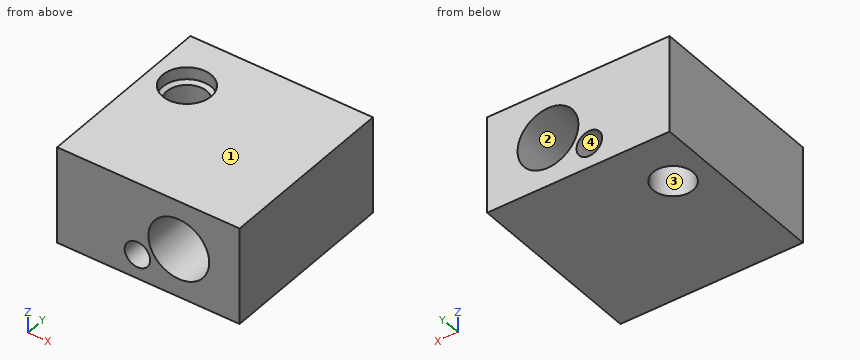
```python
from build123d import *

# Parameters (mm, degrees)
SKETCH1_W                    = 15
SKETCH1_H                    = 15
SKETCH1_R                    = 1.65
BOSS_EXTRUDE1_DEPTH          = 8
SKETCH2_R                    = 2.5
CUT_EXTRUDE1_DEPTH           = 16
SKETCH3_R                    = 1.05
CUT_EXTRUDE2_DEPTH           = 16
F_4_0_4_DIAMETER_HOLE1_D     = 4
F_4_0_4_DIAMETER_HOLE1_DEPTH = 1
F_4_0_4_DIAMETER_HOLE1_TIP   = 1.201721238


with BuildPart() as part:
    # Sketch1 → Boss-Extrude1 (new body)
    with BuildSketch(Plane.XY):
        with Locations((4.5, -3)):
            Rectangle(SKETCH1_W, SKETCH1_H)
        Circle(SKETCH1_R, mode=Mode.SUBTRACT)
    extrude(amount=BOSS_EXTRUDE1_DEPTH)

    # Sketch2 → Cut-Extrude1 (cut, through all)
    with BuildSketch(Plane.XZ.offset(10.5)):
        with Locations((7, 4)):
            Circle(SKETCH2_R)
    extrude(amount=-CUT_EXTRUDE1_DEPTH, mode=Mode.SUBTRACT)

    # Sketch3 → Cut-Extrude2 (cut, through all)
    with BuildSketch(Plane.XZ.offset(10.5)):
        with Locations((3.6, 2)):
            Circle(SKETCH3_R)
    extrude(amount=-CUT_EXTRUDE2_DEPTH, mode=Mode.SUBTRACT)

    # Ø4.0 (4) Diameter Hole1
    with Locations(Plane.XY.offset(8)):
        with Locations((0, 0)):
            Hole(F_4_0_4_DIAMETER_HOLE1_D / 2, depth=F_4_0_4_DIAMETER_HOLE1_DEPTH)
            with Locations((0, 0, -(F_4_0_4_DIAMETER_HOLE1_DEPTH + F_4_0_4_DIAMETER_HOLE1_TIP / 2))):  # 118° drill point
                Cone(0, F_4_0_4_DIAMETER_HOLE1_D / 2, F_4_0_4_DIAMETER_HOLE1_TIP, mode=Mode.SUBTRACT)


solid = part.part
```
Can you work these out from the model? Positions are in its coordinate system, mm. Face numbers are marked on the shaded views. Coordinates: 2 decimals unless noted, no trailing zeros. Loops run counter-clockwise (first coordinate to the right, second up) from the corner with the lowest first, then second, coordinate; pieces in that order, holes last.
Item 1: Suppose I cut it at C-C (z = 4). Please give me the cut outline in (x, y).
Answers below:
outline: (-3, -10.5) - (4.5, -10.5) - (4.5, 4.5) - (-3, 4.5) - close; (9.5, -10.5) - (12, -10.5) - (12, 4.5) - (9.5, 4.5) - close; hole circle Ø3.3 at (0, 0)
Item 2: Suppose I cut it at D-D (x = 7). Please give me the cut outline in (y, z), then the cut area to 3 significant figures.
Answers below:
outline: (-10.5, 0) - (4.5, 0) - (4.5, 1.5) - (-10.5, 1.5) - close; (-10.5, 6.5) - (4.5, 6.5) - (4.5, 8) - (-10.5, 8) - close
area: 45.0 mm2
Item 3: If we mould it in two halves opening along Z, with no side actions, what happens to the marked faces 1, 2, 3 and 4? For each: released by +Z, released by -Z, zero draft, split by the parting line, or undercut.
Answers below:
face 1: released by +Z
face 2: undercut
face 3: zero draft
face 4: undercut
Item 4: Suppose I cut it at B-B (z = 2). Please give me the cut outline in (x, y).
Answers below:
outline: (-3, -10.5) - (2.55, -10.5) - (2.55, 4.5) - (-3, 4.5) - close; (4.65, -10.5) - (5.5, -10.5) - (5.5, 4.5) - (4.65, 4.5) - close; (8.5, -10.5) - (12, -10.5) - (12, 4.5) - (8.5, 4.5) - close; hole circle Ø3.3 at (0, 0)
Item 5: Please list where these lines run through material, in increasing order: L1, parallel to Z at x = 3.6, y = -1.25; L2, parallel to X at y = -0.25, z = 2.5; L3, parallel to X at y = 0, z = 7.3.
Answers below:
L1: z = 0 to 0.95, 3.05 to 8
L2: x = -3 to -1.63, 1.63 to 2.68, 4.52 to 5, 9 to 12
L3: x = -3 to -2, 2 to 12
Item 6: Suppose I cut it at A-A (y = 0). Please give me the cut outline in (x, z).
Answers below:
outline: (-3, 0) - (-1.65, 0) - (-1.65, 6.79) - (-2, 7) - (-2, 8) - (-3, 8) - close; (1.65, 0) - (12, 0) - (12, 8) - (2, 8) - (2, 7) - (1.65, 6.79) - close; hole circle Ø2.1 at (3.6, 2); hole circle Ø5 at (7, 4)
